from build123d import *

# Parameters (mm, degrees)
SKETCH2_W           = 101.6
SKETCH2_H           = 101.6
BOSS_EXTRUDE2_DEPTH = 5
SKETCH3_W           = 5
SKETCH3_H           = 50.8
BOSS_EXTRUDE3_DEPTH = 25.4
SKETCH4_W           = 5
SKETCH4_H           = 50.8
BOSS_EXTRUDE4_DEPTH = 25.4
SKETCH8_R           = 3.556
CUT_EXTRUDE1_DEPTH  = 135.392047756
CUT_EXTRUDE2_REACH  = 136.392
SKETCH9_R           = 0.762
SKETCH11_R          = 7.9502
CUT_EXTRUDE3_DEPTH  = 146.911891222
CUT_EXTRUDE5_REACH  = 136.392
SKETCH18_R          = 0.762
SKETCH19_W          = 22.350467385
SKETCH19_H          = 21.198381437
BOSS_EXTRUDE5_DEPTH = 76.2
SKETCH22_R          = 5
CUT_EXTRUDE6_DEPTH  = 179.909697893


with BuildPart() as part:
    # Sketch2 → Boss-Extrude2 (new body)
    with BuildSketch(Plane(origin=(0, 0, 0), x_dir=(1, 0, 0), z_dir=(0, 1, 0))):
        with Locations((50.8, -50.8)):
            Rectangle(SKETCH2_W, SKETCH2_H)
    extrude(amount=BOSS_EXTRUDE2_DEPTH)

    # Sketch3 → Boss-Extrude3 (add)
    with BuildSketch(Plane(origin=(0, 5, 0), x_dir=(1, 0, 0), z_dir=(0, 1, 0))):
        with Locations((21.55, -50.8)):
            Rectangle(SKETCH3_W, SKETCH3_H)
    extrude(amount=BOSS_EXTRUDE3_DEPTH)

    # Sketch4 → Boss-Extrude4 (add)
    with BuildSketch(Plane(origin=(0, 5, 0), x_dir=(1, 0, 0), z_dir=(0, 1, 0))):
        with Locations((80.05, -50.8)):
            Rectangle(SKETCH4_W, SKETCH4_H)
    extrude(amount=BOSS_EXTRUDE4_DEPTH)

    # Sketch8 → Cut-Extrude1 (cut, through all)
    with BuildSketch(Plane.ZY.offset(-19.05)):
        with Locations((50.8, 23.542)):
            Circle(SKETCH8_R)
    extrude(amount=-CUT_EXTRUDE1_DEPTH, mode=Mode.SUBTRACT)

    # Sketch9 → Cut-Extrude2 (cut, up to next)
    with BuildSketch(Plane(origin=(82.55, 0, 0), x_dir=(0, 0, -1), z_dir=(1, 0, 0)), mode=Mode.PRIVATE) as cut_extrude2_sk1:
        with Locations((-50.8, 12.62)):
            Circle(SKETCH9_R)
    cut_extrude2_tool1 = extrude(cut_extrude2_sk1.sketch, amount=-CUT_EXTRUDE2_REACH, mode=Mode.PRIVATE) & part.part
    add(cut_extrude2_tool1.solids().sort_by_distance((82.55, 12.62, 50.8))[0], mode=Mode.SUBTRACT)

    # Sketch11 → Cut-Extrude3 (cut, through all)
    with BuildSketch(Plane(origin=(0, 5, 0), x_dir=(1, 0, 0), z_dir=(0, 1, 0))):
        with Locations(Location((59.61, -50.8, 0), (0, 0, 270))):
            Circle(SKETCH11_R)
    extrude(amount=-CUT_EXTRUDE3_DEPTH, mode=Mode.SUBTRACT)

    # Sketch18 → Cut-Extrude5 (cut, up to next)
    with BuildSketch(Plane.ZY.offset(-19.05), mode=Mode.PRIVATE) as cut_extrude5_sk1:
        with Locations(Location((50.8, 12.62, 0), (0, 0, 180))):
            Circle(SKETCH18_R)
    cut_extrude5_tool1 = extrude(cut_extrude5_sk1.sketch, amount=-CUT_EXTRUDE5_REACH, mode=Mode.PRIVATE) & part.part
    add(cut_extrude5_tool1.solids().sort_by_distance((19.05, 12.62, 50.8))[0], mode=Mode.SUBTRACT)

    # Sketch19 → Boss-Extrude5 (add)
    with BuildSketch(Plane.XZ):
        with Locations((59.324658632, 50.761526183)):
            Rectangle(SKETCH19_W, SKETCH19_H)
    extrude(amount=BOSS_EXTRUDE5_DEPTH)

    # Sketch22 → Cut-Extrude6 (cut, through all)
    with BuildSketch(Plane.XZ.offset(76.2)):
        with Locations(Location((59.61, 50.8, 0), (0, 0, 270))):
            Circle(SKETCH22_R)
    extrude(amount=-CUT_EXTRUDE6_DEPTH, mode=Mode.SUBTRACT)


solid = part.part
Work out the finished part from the listing and answer in its coordinate system (mm). A direction names the side the tool comes from. Round coordinates to 2 decimals unless told otherwise and drop trailing zeros. Write each loop counter-clockwise with the first axis right and the second up, starting at its lowest first coordinate (ties: lowest second). Pieces come first, ordered by that corner, then holes. Notation, with made-up numbers: (9, 32) - (25, 32) arc R26 cw to (25, 55) - close; hole circle Ø3 at (54.5, 19). An arc over 180 degrees is marked (long way). Answer in a Markdown table with one row per item. Add a question column.
1. Given pin 1 (1 mm diameter, centred on x = 91, z = 33, fed in from -Y); pin 2 (6.5 mm diameter, centred on y = -47, z = 48, fed in from -X); pin 3 (11 mm diameter, centred on x = 55, y = -54.5, fed in from -Z); pin 4 (1.2 mm diameter, centred on y = 12.62, z = 50.8, fed in from -X), each flat-ended and moving along its own axis, determine where each tip first touches the part or whether it passes through.
2. For faces 4 (the flat face through (82.55, 18, 51)), 5 (the flat face through (70.5, -38, 51)), 6 (the flat face through (48.149, -38, 51)), 7 (the flat face through (59, -38, 61.361)), determine the directions among +Z, -Z, +X, -X, +Y, -Y from which every point of the face is accessible in a straight line to the end or side of a thin tool.
3. Find the intervals of material crossed by line 1 along Y through (x, z) = (21.55, 50.8); line 2 along X through (y, z) = (14.5, 29); line 3 along Z through (x, y) = (23, 14), in increasing order. Write a range as from..to.
4. A cutting plane is placed at C-C, the plane x = 94.5. Determine the outline of the cut face in (y, z), and give its area (3 significant figures).
5. A cutting plane is placed at D-D, the plane z = 9. Determine the outline of the cut face in (x, y).
6. The mould has two halves that part along Z. Classify faces 1 (the flat face through (50, 2, 101.6)), 2 (the cylindrical face through (55.174, -38.633, 48.493)), 3 (the flat face through (0, 2, 52)): +Z half, -Z half, draft (parallel to the pull), parting line (faces both ways), or undercut.
7. A cutting plane is placed at A-A, the plane x = 59.61. Determine the outline of the cut face in (y, z).
8. A cutting plane is placed at B-B, the plane y = -15. Determine the outline of the cut face in (x, z).
Worked out:
| question | item | result |
|---|---|---|
| 1 | pin 1 | y = 0 |
| 1 | pin 2 | x = 48.15 |
| 1 | pin 3 | z = 40.16 |
| 1 | pin 4 | through |
| 2 | face 4 | +Z, -Z, +X, +Y |
| 2 | face 5 | +Z, -Z, +X, -Y |
| 2 | face 6 | +Z, -Z, -X, -Y |
| 2 | face 7 | +Z, +X, -X, -Y |
| 3 | line 1 | 0..11.86, 13.38..19.99, 27.1..30.4 |
| 3 | line 2 | 19.05..24.05, 77.55..82.55 |
| 3 | line 3 | 25.4..76.2 |
| 4 | outline | (0, 0) - (5, 0) - (5, 101.6) - (0, 101.6) - close |
| 4 | area | 508 mm^2 |
| 5 | outline | (0, 0) - (101.6, 0) - (101.6, 5) - (0, 5) - close |
| 6 | face 1 | +Z half |
| 6 | face 2 | undercut |
| 6 | face 3 | draft |
| 7 | outline | (-76.2, 40.16) - (0, 40.16) - (0, 0) - (5, 0) - (5, 42.85) - (0, 42.85) - (0, 45.8) - (-76.2, 45.8) - close; (-76.2, 55.8) - (0, 55.8) - (0, 58.75) - (5, 58.75) - (5, 101.6) - (0, 101.6) - (0, 61.36) - (-76.2, 61.36) - close |
| 8 | outline | (48.15, 40.16) - (70.5, 40.16) - (70.5, 61.36) - (48.15, 61.36) - close; hole circle Ø10 at (59.61, 50.8) |
